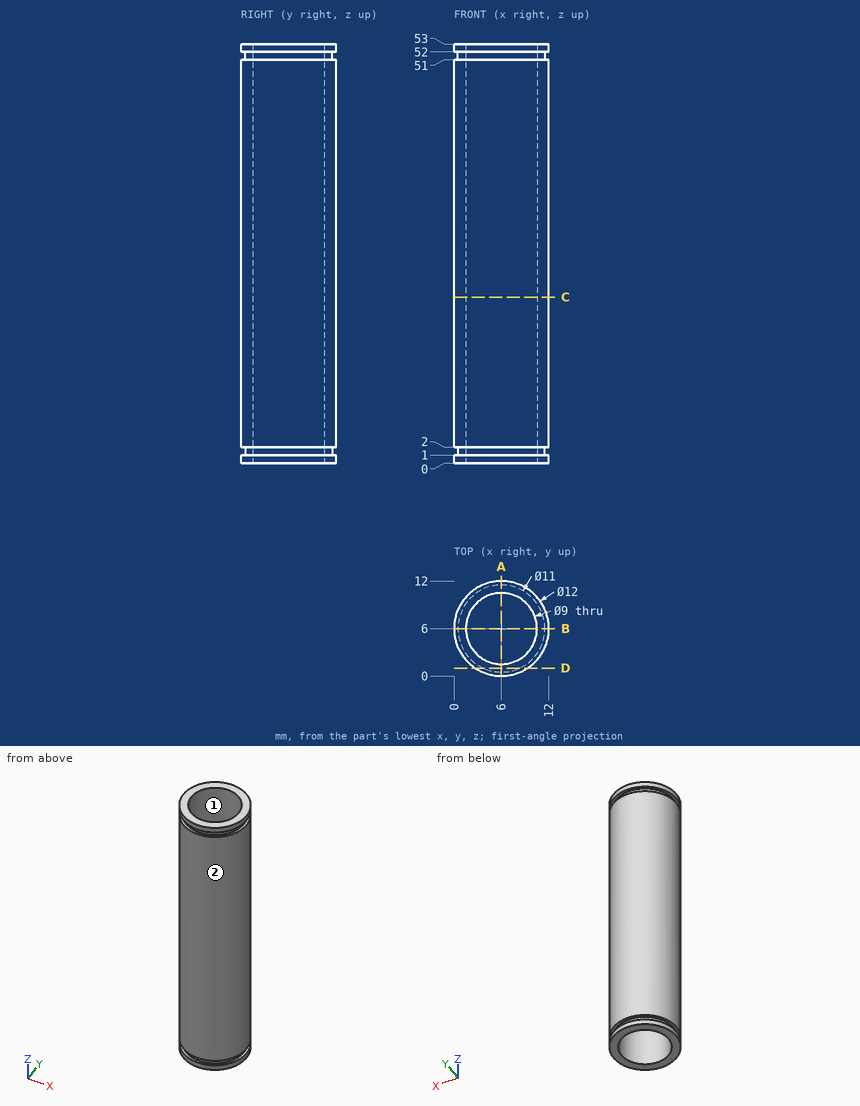
The figure shows three views and two pictorial views of one solid part (mm, origin at its lowest corner). Answer the questions. Coordinates: 2 decimals unless noted, no trailing zeros. Loops run counter-clockwise (first coordinate to the right, second up) from the corner with the lowest first, then second, coordinate; pieces in that order, holes last. Notation, with made-up numbers: (-37.5, 29) -> (20.5, 29) arc R15 ccw to (20.5, 49) -> close; hole circle Ø3 at (-2, 52.25). An arc over 180 degrees is marked (long way). Return JSON: item names as keys, results as strings. Group by question number.
(1) A cutting plane is placed at A-A on x = 6. Write down the section's boundary in (y, z).
(2) Given pin 1 Ø1 at (y, z) = (2.5, 40.5) entering from +X, flat-ended and moving along its own axis, determine where the tip first touches the part or whether it passes through.
(3) Determine the mould class of the marked faces 1 and 2 for opening direction Y: released by +Y, released by -Y, zero draft, split by the parting line, or undercut.
(4) A cutting plane is placed at C-C on z = 21. Write down the section's boundary in (x, y), and give its area (3 significant figures).
(5) Find the intervals of material crossed by probe 1 along Z at (x, y) = (3.75, 11.25); probe 2 along Y at (x, z) = (6, 40.5); probe 3 along Y at (x, z) = (2.5, 17), in increasing order. Write a range as from..to.
(6) A cutting plane is placed at D-D on y = 1. Write down the section's boundary in (x, z), and give its area (3 significant figures).
The answers:
{
 "1": {"outline": "(0, 0) -> (1.5, 0) -> (1.5, 53) -> (0, 53) -> (0, 52) -> (0.5, 52) -> (0.5, 51) -> (0, 51) -> (0, 2) -> (0.5, 2) -> (0.5, 1) -> (0, 1) -> close; (10.5, 0) -> (12, 0) -> (12, 1) -> (11.5, 1) -> (11.5, 2) -> (12, 2) -> (12, 51) -> (11.5, 51) -> (11.5, 52) -> (12, 52) -> (12, 53) -> (10.5, 53) -> close"},
 "2": {"pin 1": "stops at x = 11.2"},
 "3": {"face 1": "undercut", "face 2": "split by the parting line"},
 "4": {"outline": "circle Ø12 at (6, 6); hole circle Ø9 at (6, 6)", "area": "49.5 mm^2"},
 "5": {"probe 1": "z = 0..1, 2..51, 52..53", "probe 2": "y = 0..1.5, 10.5..12", "probe 3": "y = 1.13..3.17, 8.83..10.87"},
 "6": {"outline": "(2.68, 0) -> (9.32, 0) -> (9.32, 1) -> (8.29, 1) -> (8.29, 2) -> (9.32, 2) -> (9.32, 51) -> (8.29, 51) -> (8.29, 52) -> (9.32, 52) -> (9.32, 53) -> (2.68, 53) -> (2.68, 52) -> (3.71, 52) -> (3.71, 51) -> (2.68, 51) -> (2.68, 2) -> (3.71, 2) -> (3.71, 1) -> (2.68, 1) -> close", "area": "347 mm^2"}
}
